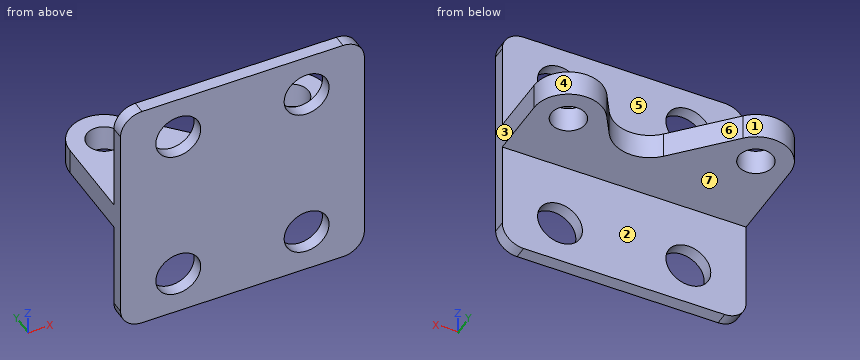
from build123d import *

# Parameters (mm, degrees)
EXTRUDE_1_DEPTH      = 3
EXTRUDE_1_DEPTH_BACK = 3
SKETCH_1_R           = 4
SKETCH_2_R           = 5.25
EXTRUDE_2_DEPTH      = 3


with BuildPart() as part:
    # Sketch 1 → Extrude 1 (new, two sides: drawn at the far end of the back side and taken through both)
    with BuildSketch(Plane.XY.offset(-EXTRUDE_1_DEPTH_BACK)):
        with BuildLine():
            Line((0, 0), (57, 0))
            Line((57, 0), (57, 17.5))
            ThreePointArc((57, 17.5), (51.229837516, 25.182956765), (42.243043837, 21.782936307))
            Line((42.243043837, 21.782936307), (39.179265923, 16.949380174))
            ThreePointArc((39.179265923, 16.949380174), (32.794593586, 13.037221435), (25.793283338, 15.692533403))
            Line((25.793283338, 15.692533403), (13.841615682, 28.465850915))
            ThreePointArc((13.841615682, 28.465850915), (5.061711847, 30.44086438), (0, 23))
            Line((0, 23), (0, 0))
        make_face()
        with Locations((49, 17.5)):
            Circle(SKETCH_1_R, mode=Mode.SUBTRACT)
        with Locations((8, 23)):
            Circle(SKETCH_1_R, mode=Mode.SUBTRACT)
    extrude(amount=EXTRUDE_1_DEPTH + EXTRUDE_1_DEPTH_BACK)

    # Sketch 2 → Extrude 2 (add)
    with BuildSketch(Plane(origin=(0, 0, 0), x_dir=(1, 0, 0), z_dir=(0, 1, 0))):
        with BuildLine():
            Line((5, -28.5), (52, -28.5))
            ThreePointArc((52, -28.5), (55.535533906, -27.035533906), (57, -23.5))
            Line((57, -23.5), (57, 23.5))
            ThreePointArc((57, 23.5), (55.535533906, 27.035533906), (52, 28.5))
            Line((52, 28.5), (5, 28.5))
            ThreePointArc((5, 28.5), (1.464466094, 27.035533906), (0, 23.5))
            Line((0, 23.5), (0, -23.5))
            ThreePointArc((0, -23.5), (1.464466094, -27.035533906), (5, -28.5))
        make_face()
        with Locations(Location((43.5, -18.5, 0), (0, 0, 270))):
            Circle(SKETCH_2_R, mode=Mode.SUBTRACT)
        with Locations(Location((43.5, 18.5, 0), (0, 0, 270))):
            Circle(SKETCH_2_R, mode=Mode.SUBTRACT)
        with Locations(Location((13.5, -18.5, 0), (0, 0, 270))):
            Circle(SKETCH_2_R, mode=Mode.SUBTRACT)
        with Locations(Location((13.5, 18.5, 0), (0, 0, 270))):
            Circle(SKETCH_2_R, mode=Mode.SUBTRACT)
    extrude(amount=EXTRUDE_2_DEPTH)


solid = part.part
Geometry: final body of the model. Coordinates: model frame, mm. Face numbers are marked on the shaded views. A direction names the side the tool comes from. Give positions to 0.01 mm unless a question says otherwise; leave off trailing zeros. Write each loop counter-clockwise with the first axis right and the second up, starting at its lowest first coordinate (ties: lowest second). Pieces come first, ordered by that corner, then holes. Notation, with made-up numbers: (77, 79.25) - (119, 79.25) arc R5 cw to (119, 87.25) - close; hole circle Ø9 at (36.25, 36). An arc over 180 degrees is marked (long way). Return JSON: item names as keys, results as strings. Group by question number.
1) Section D-D on x = 43.5. Return the cut outline in (y, z).
2) Section C-C on x = 9. Return the cut outline in (y, z).
3) Line query: line 1 (Z direction, x = 18, y = 8.5); line 2 (Y direction, x = 24, z = -12); line 3 (Y direction, x = 40, z = -2.5). Output: solid intervals per line, ascending.
4) Set-up query: the marked faces 5, 6 and 7. Return all of +Z, -Z, +X, -X, +Y, -Y with unobstructed straight access to the full face (end or side cutting, diameter ignored); none if empty.
5) Mould query, pull axis X, two halves, no side actions, for the marked faces 1, 2, 3 and 4. Classes: released by +X, released by -X, zero draft, split by the parting line, or undercut.
6) Section A-A on z = -18.5. Return the cut outline in (x, y).
7) Section B-B on x = 28. Return the cut outline in (y, z).
8) First-contact query: P1, Ø6.5, axis at x = 13.5, z = -18.5, coming from the +Y side; P2, Ø2, axis at x = 14.5, y = 22.5, coming from the +Z side; P3, Ø12, axis at x = 50.5, y = 20.5, coming from the -Z side; P4, Ø13, axis at x = 14.5, z = 10, coming from the +Y side. Flat tips, straight axial feed; report the tip coordinate or a pass-through.
Filled in:
{
 "1": {"outline": "(0, -28.5) - (3, -28.5) - (3, -23.75) - (0, -23.75) - close; (0, -13.25) - (3, -13.25) - (3, -3) - (23.31, -3) - (23.31, 3) - (3, 3) - (3, 13.25) - (0, 13.25) - close; (0, 23.75) - (3, 23.75) - (3, 28.5) - (0, 28.5) - close"},
 "2": {"outline": "(0, -28.5) - (3, -28.5) - (3, -21.2) - (0, -21.2) - close; (0, -15.8) - (3, -15.8) - (3, -3) - (19.13, -3) - (19.13, 3) - (3, 3) - (3, 15.8) - (0, 15.8) - close; (0, 21.2) - (3, 21.2) - (3, 28.5) - (0, 28.5) - close; (26.87, -3) - (30.94, -3) - (30.94, 3) - (26.87, 3) - close"},
 "3": {"line 1": "z = -3 to 3", "line 2": "y = 0 to 3", "line 3": "y = 0 to 18.24"},
 "4": {"face 5": "+Z, +X, -X, +Y", "face 6": "+Z, -Z, +Y", "face 7": "-Z, +X, -X, +Y"},
 "5": {"face 1": "split by the parting line", "face 2": "zero draft", "face 3": "released by +X", "face 4": "undercut"},
 "6": {"outline": "(0, 0) - (8.25, 0) - (8.25, 3) - (0, 3) - close; (18.75, 0) - (38.25, 0) - (38.25, 3) - (18.75, 3) - close; (48.75, 0) - (57, 0) - (57, 3) - (48.75, 3) - close"},
 "7": {"outline": "(0, -28.5) - (3, -28.5) - (3, -3) - (14, -3) - (14, 3) - (3, 3) - (3, 28.5) - (0, 28.5) - close"},
 "8": {"P1": "passes through", "P2": "stops at z = 3", "P3": "stops at z = -3", "P4": "stops at y = 3"}
}
